CAD build for the part. Positions are in the model's coordinates, mm. Face numbers are marked on the shaded views. A direction names the side the tool comes from. Coordinates: 2 decimals unless noted, no trailing zeros. Loops run counter-clockwise (first coordinate to the right, second up) from the corner with the lowest first, then second, coordinate; pieces in that order, holes last. Notation, with made-up numbers: (69.25, -13.5) -> (121.25, -13.5) arc R27 ccw to (121.25, 22.5) -> close; hole circle Ø1 at (68, -17). An arc over 180 degrees is marked (long way). Return JSON: item names as keys, results as strings. Group by question number.
(1) Probe L1, parallel to Y at x = -4.5, z = 5; L2, parallel to Y at x = 0.5, z = 2; L3, parallel to Z at x = -11, y = -21. List the from-to ranges inside material, lowest first.
(2) Tool access for the marked faces 1, 2 and 3: list every direction of +Z, -Z, +X, -X, +Y, -Y with a clear straight run to the whole face (end or side of a thin tool).
(3) Saw through at D-D on z = -9. Write the cut outline in (x, y).
(4) Saw through at C-C on y = -21. Write the cut outline in (x, z).
(5) Flat gauge pins, fed straight in: pin 1 Ø8.5 at (x, y) = (-7.5, 3) entering from -Z; pin 2 Ø2 at (y, z) = (4, 0.5) entering from +X; pin 3 Ø10 at (x, y) = (7.5, -21.5) entering from -Z. Where does each tip first touch, or does it go through?
(6) Saw through at B-B on z = -1. Write the cut outline in (x, y), then the cut area to 3 significant figures.
(7) Saw through at A-A on x = 0. Write the cut outline in (y, z), then the cut area to 3 significant figures.
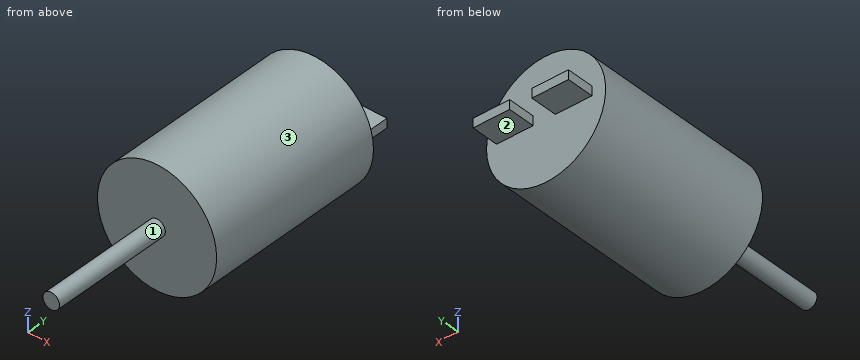
```python
from build123d import *

# Parameters (mm, degrees)
F0_R     = 16.51
F1_DEPTH = 50.8
F2_R     = 2.286
F3_DEPTH = 34.29
F4_W     = 10.16
F4_H     = 2.54
F5_DEPTH = 7.62


with BuildPart() as f1:
    # F0 (on Front) → F1 (new body)
    with BuildSketch(Plane.XZ):
        Circle(F0_R)
    extrude(amount=F1_DEPTH)

    # F2 (on face) → F3 (join)
    with BuildSketch(Plane.XZ.offset(50.8)):
        Circle(F2_R)
    extrude(amount=F3_DEPTH)

    # F4 (on face) → F5 (join)
    with BuildSketch(Plane(origin=(0, 0, 0), x_dir=(-1, 0, 0), z_dir=(0, 1, 0))):
        with Locations((-8.658255, 1.27)):
            Rectangle(F4_W, F4_H)
        with Locations((7.64519, 1.27)):
            Rectangle(F4_W, F4_H)
    extrude(amount=F5_DEPTH)


solid = f1.part
```
Geometry results:
{
 "1": {"L1": "-50.8 to 0", "L2": "-85.09 to 0", "L3": "-12.31 to 12.31"},
 "2": {"face 1": "-Y", "face 2": "-Z, +X, -X, +Y", "face 3": "+Y, -Y"},
 "3": {"outline": "(-13.84, -50.8) -> (13.84, -50.8) -> (13.84, 0) -> (-13.84, 0) -> close"},
 "4": {"outline": "circle Ø33.02 at (0, 0)"},
 "5": {"pin 1": "z = -15.89", "pin 2": "x = 13.74", "pin 3": "z = -16.32"},
 "6": {"outline": "(-16.48, -50.8) -> (-2.06, -50.8) -> (-2.06, -85.09) -> (2.06, -85.09) -> (2.06, -50.8) -> (16.48, -50.8) -> (16.48, 0) -> (-16.48, 0) -> close", "area": "1,820 mm²"},
 "7": {"outline": "(-85.09, -2.29) -> (-50.8, -2.29) -> (-50.8, -16.51) -> (0, -16.51) -> (0, 16.51) -> (-50.8, 16.51) -> (-50.8, 2.29) -> (-85.09, 2.29) -> close", "area": "1,830 mm²"}
}
